Check sheet for the modelled part. Datum: model origin and axes. Units: mm. Face numbers are marked on the shaded views. A direction names the side the tool comes from. Coordinates: 2 decimals unless noted, no trailing zeros. Write each loop counter-clockwise with the first axis right and the second up, starting at its lowest first coordinate (ties: lowest second). Pieces come first, ordered by that corner, then holes. Notation, with made-up numbers: (13, 11) -> (66, 11) arc R14 cw to (66, 36) -> close; hole circle Ø4 at (22.5, 9). An arc over 180 degrees is marked (long way). Put each result on its own line as item: value.
Autodesk Inventor part; units mm, degrees
ref_plane "YZ Plane" through (0, 0, 0) normal (1, 0, 0) x (0, 1, 0)
ref_plane "XZ Plane" through (0, 0, 0) normal (0, 1, 0) x (-1, 0, 0)
ref_plane "XY Plane" through (0, 0, 0) normal (0, 0, 1) x (1, 0, 0)
sketch "Sketch1" plane through (0, 0, 0) normal (0, 1, 0) x (-1, 0, 0)
  circle A0 centre (0, 0) radius 47.5
  line L0 (-25, 15) -> (25, 15)
  line L1 (25, 15) -> (25, -15)
  line L2 (25, -15) -> (-25, -15)
  line L3 (-25, -15) -> (-25, 15)
  line L4 (-25, 15) -> (25, -15) construction
  line L5 (25, 15) -> (-25, -15) construction
  line L6 (-26.25, 26.25) -> (26.25, 26.25) construction
  line L7 (26.25, 26.25) -> (26.25, -26.25) construction
  line L8 (26.25, -26.25) -> (-26.25, -26.25) construction
  line L9 (-26.25, -26.25) -> (-26.25, 26.25) construction
  line L10 (-26.25, 26.25) -> (26.25, -26.25) construction
  line L11 (26.25, 26.25) -> (-26.25, -26.25) construction
  dimension "d0" = 30
  dimension "d2" = 95
  dimension "holeL" = 52.5
  dimension "d27" = 50
extrude "Extrusion1" add sketch "Sketch1" against normal blind 57 contours A0 | L0 L1 L2 L3
extrude "Extrusion2" cut sketch "Sketch1" against normal blind 23 contours L0 L1 L2 L3
sketch "Sketch3" plane through (0, 0, 0) normal (0, 1, 0) x (1, 0, 0)
  line L0 (-25, -15) -> (-25, 15) construction
  line L1 (-25, 15) -> (25, 15) construction
  line L2 (25, 15) -> (25, -15) construction
  line L3 (25, -15) -> (-25, -15) construction
  circle A0 centre (0, 0) radius 47.5 construction
  circle A1 centre (18.8128, 8.8128) radius 8.75
  line L4 (18.8128, 8.8128) -> (25, 15) construction
  line L5 (-66.5, 0) -> (66.5, 0) construction
  line L6 (0, 66.5) -> (0, -66.5) construction
  circle A2 centre (18.8128, -8.8128) radius 8.75
  circle A3 centre (-18.8128, 8.8128) radius 8.75
  circle A4 centre (-18.8128, -8.8128) radius 8.75
  dimension "d34" = 17.5
  dimension "d33" = 45
extrude "Extrusion3" cut sketch "Sketch3" against normal up to surface (23 mm away)
hole "Hole1" at (-26.25, 0, -26.25) at (26.25, 0, -26.25) at (26.25, 0, 26.25) at (-26.25, 0, 26.25) direction (0, -1, 0) diameter 6.647 depth 17 tip angle 118 countersink diameter 10 countersink angle 90
chamfer "Chamfer1" distance 1 angle 45 8 edges at (0, 0, -15) (25, 0, 0) (0, 0, 15) (-25, 0, 0) (-25, 0, -15) (-25, 0, 15) (25, 0, -15) (25, 0, 15)
chamfer "Chamfer2" distance 2 angle 45 1 edges at (47.5, -57, 0)
sketch "Sketch2" plane through (0, -57, 0) normal (0, -1, 0) x (1, 0, 0)
  circle A0 centre (0, 0) radius 15 construction
  circle A1 centre (0, 0) radius 19 construction
  dimension "d23" = 4
  dimension "d24" = 30
mark "Mark1"
properties part number "HM1_FIXT1-001"
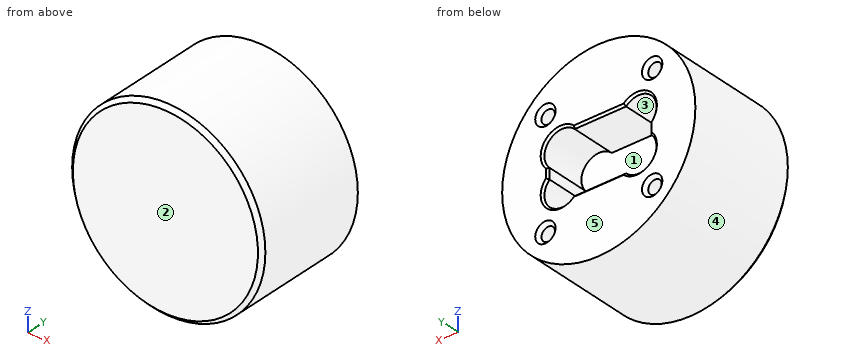
Q1. Depth check by flat-ended pin: P1, Ø17.5, axis at x = 3, y = -12.5, coming from the +Z side; P2, Ø1, axis at x = 15, y = -30, coming from the -Z side; P3, Ø17.5, axis at x = -2.5, z = 4, coming from the +Y side. Enter the tip coordinate at first touch or a pass-through.
Recorded:
P1: stops at z = 47.5
P2: stops at z = -45.23
P3: stops at y = -23
Q2. Cross-section at A-A (x = 0). Record the cut outline in (y, z), plus the area to 3 significant figures.
Recorded:
outline: (-57, -45.5) -> (-55, -47.5) -> (0, -47.5) -> (0, -16) -> (-1, -15) -> (-23, -15) -> (-23, 15) -> (-1, 15) -> (0, 16) -> (0, 47.5) -> (-55, 47.5) -> (-57, 45.5) -> close
area: 4,720 mm2
Q3. Tool access check on the marked faces 1 and 2. Record the directions out of +Z, -Z, +X, -X, +Y, -Y that give a thin tool (end or side, any length) a straight path to the whole face; none if there is none.
Recorded:
face 1: +Y
face 2: +Z, -Z, +X, -X, -Y
Q4. Cross-section at B-B (z = 0). Record the cut outline in (x, y).
Recorded:
outline: (-47.5, -55) -> (-45.5, -57) -> (45.5, -57) -> (47.5, -55) -> (47.5, 0) -> (26, 0) -> (25, -1) -> (25, -23) -> (-25, -23) -> (-25, -1) -> (-26, 0) -> (-47.5, 0) -> close
Q5. Material ranges on line 1 along Z through (x, y) = (26.25, -6.75); line 2 along X through (y, z) = (-10.5, 26.25); line 3 along X through (y, z) = (-13, -26), recorded low to high.
Recorded:
line 1: z = -39.59 to -29.57, -22.93 to -13.42, -4.2 to 4.2, 13.42 to 22.93, 29.57 to 39.59
line 2: x = -39.59 to -29.57, -22.93 to 22.93, 29.57 to 39.59
line 3: x = -39.75 to -29.56, -22.94 to 22.94, 29.56 to 39.75
Q6. Cross-section at C-C (y = -29). Record the cut outline in (x, z).
Recorded:
outline: circle Ø95 at (0, 0)
Q7. Mould release check, pull along X, two halves, no side actions. Record for the marked faces 3, 4 and 5: released by +X, released by -X, zero draft, split by the parting line, or undercut.
Recorded:
face 3: undercut
face 4: split by the parting line
face 5: zero draft
